```python
from build123d import *

# Parameters (mm, degrees)
F0_W     = 50
F0_H     = 100
F1_DEPTH = 50
F2_D     = 26
F3_D     = 6.6
F4_D     = 13.2
F5_R     = 5
F7_D     = 4.2
F7_DEPTH = 52.4
F7_TIP   = 1.2618073
F8_D     = 4.2
F8_DEPTH = 50
F8_TIP   = 1.2618073


with BuildPart() as f1:
    # F0 (on Front) → F1 (new body)
    with BuildSketch(Plane.XZ):
        Rectangle(F0_W, F0_H)
    extrude(amount=F1_DEPTH)

    # F2 (through all)
    with Locations(Plane(origin=(0, 0, 0), x_dir=(1, 0, 0), z_dir=(0, 1, 0))):
        with Locations((0, -25), (0, 25)):
            Hole(F2_D / 2)

    # F3 (through all)
    with Locations(Plane(origin=(0, 0, 0), x_dir=(1, 0, 0), z_dir=(0, 1, 0))):
        with Locations((14.5, 0)):
            Hole(F3_D / 2)

    # F4 (through all)
    with Locations(Plane(origin=(0, 0, 0), x_dir=(1, 0, 0), z_dir=(0, 1, 0))):
        with Locations((-13, 0)):
            Hole(F4_D / 2)

    # F5
    f5_edges = [f1.edges().sort_by_distance(p)[0] for p in [
        (-25, -25, 50),
        (25, -25, 50),
        (25, -25, -50),
        (-25, -25, -50),
    ]]
    fillet(f5_edges, radius=F5_R)

    # F7
    with Locations(Plane(origin=(-25, 0, 0), x_dir=(0, -1, 0), z_dir=(-1, 0, 0))):
        with Locations((12, 0), (38, 0)):
            Hole(F7_D / 2, depth=F7_DEPTH)
            with Locations((0, 0, -(F7_DEPTH + F7_TIP / 2))):  # 118° drill point
                Cone(0, F7_D / 2, F7_TIP, mode=Mode.SUBTRACT)

    # F8
    with Locations(Plane(origin=(-25, 0, 0), x_dir=(0, -1, 0), z_dir=(-1, 0, 0))):
        with Locations((12, -26), (38, -26)):
            Hole(F8_D / 2, depth=F8_DEPTH)
            with Locations((0, 0, -(F8_DEPTH + F8_TIP / 2))):  # 118° drill point
                Cone(0, F8_D / 2, F8_TIP, mode=Mode.SUBTRACT)


solid = f1.part
```
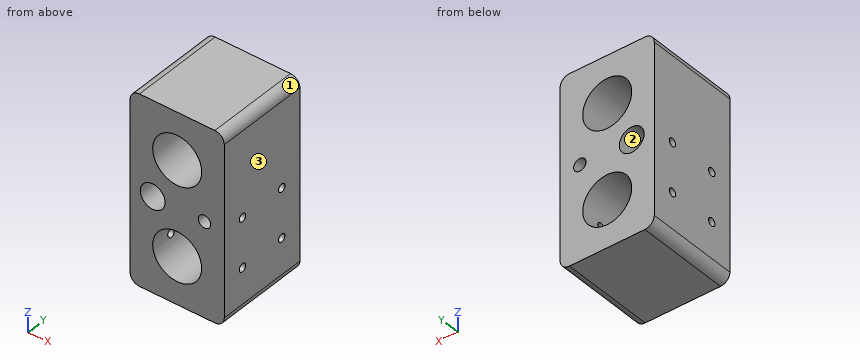
Could you check a few things on this model? Use its own coordinates, in mm. Face numbers are marked on the shaded views. Coordinates: 2 decimals unless noted, no trailing zeros. Loops run counter-clockwise (first coordinate to the right, second up) from the corner with the lowest first, then second, coordinate; pieces in that order, holes last.
1) Imagine slicing it at A-A (x = 0). List the corners of the cut face in (y, z) for me.
Reported:
outline: (-50, -50) - (0, -50) - (0, -38) - (-50, -38) - close; (-50, -12) - (0, -12) - (0, 12) - (-50, 12) - close; (-50, 38) - (0, 38) - (0, 50) - (-50, 50) - close; hole circle Ø4.2 at (-38, 0); hole circle Ø4.2 at (-12, 0)
2) Thinking about a two-plate mould opening in Z: for the marked faces 1, 2 and 3, which applies, released by +Z, released by -Z, zero draft, split by the parting line, or undercut?
Reported:
face 1: released by +Z
face 2: undercut
face 3: zero draft
3) Imagine slicing it at D-D (y = -45). List the corners of the cut face in (x, z) for me.
Reported:
outline: (-25, -45) arc R5 ccw to (-20, -50) - (20, -50) arc R5 ccw to (25, -45) - (25, 45) arc R5 ccw to (20, 50) - (-20, 50) arc R5 ccw to (-25, 45) - close; hole circle Ø13.2 at (-13, 0); hole circle Ø26 at (0, -25); hole circle Ø26 at (0, 25); hole circle Ø6.6 at (14.5, 0)
4) Imagine slicing it at B-B (x = 14.5). List the corners of the cut face in (y, z) for me.
Reported:
outline: (-50, -50) - (0, -50) - (0, -3.3) - (-50, -3.3) - close; (-50, 3.3) - (0, 3.3) - (0, 50) - (-50, 50) - close; hole circle Ø4.2 at (-38, -26); hole circle Ø4.2 at (-12, -26)
5) Will this pin go through, and if not, where does the flat tip stop? pin 1 Ø23.5 at (x, z) = (0, 25) entering from +Y.
Reported:
pin 1: passes through
6) Imagine slicing it at C-C (z = -26). List the corners of the cut face in (x, y) for me, and give its area (3 significant figures).
Reported:
outline: (-25, -50) - (-12.96, -50) - (-12.96, -40.1) - (-25, -40.1) - close; (-25, -35.9) - (-12.96, -35.9) - (-12.96, -14.1) - (-25, -14.1) - close; (-25, -9.9) - (-12.96, -9.9) - (-12.96, 0) - (-25, 0) - close; (12.96, -50) - (25, -50) - (25, -40.1) - (12.96, -40.1) - close; (12.96, -35.9) - (25, -35.9) - (25, -14.1) - (12.96, -14.1) - close; (12.96, -9.9) - (25, -9.9) - (25, 0) - (12.96, 0) - close
area: 1,000 mm2
7) Please list where these lines run through material, in increasing order: line 1 along Z through (x, y) = (-0.5, -7.5); line 2 along Z through (x, y) = (20, -12); line 3 along Y through (x, z) = (2.75, 0).
Reported:
line 1: z = -50 to -37.99, -12.01 to 12.01, 37.99 to 50
line 2: z = -50 to -28.1, -23.9 to -2.1, 2.1 to 50
line 3: y = -50 to -40.1, -35.9 to -14.1, -9.9 to 0
